Input: part model. Units: mm. Frame: model coordinates. Face numbers are marked on the shaded views. A direction names the side the tool comes from. Coordinates: 2 decimals unless noted, no trailing zeros. Order: outer loops, then holes, each group sorted by start corner. A loop starts at its lowest first (then second) coordinate and runs counter-clockwise, first axis right, second up. Notation, with made-up numbers: M -22,-2.75 L 35,-2.75 A17 cw 35,13.25 Z; hole C 36,-21 d6. An arc over 180 degrees is marked long. One line per item, written item: value.
Solid Edge part; units mm, degrees
sketch "Sketch1" plane through (0, 0, 0) normal (0, -1, 0) x (1, 0, 0)
  line L0 (7.5, -37.5) -> (-7.5, -37.5)
  line L1 (-7.5, -37.5) -> (-7.5, 47.5)
  line L2 (-7.5, 47.5) -> (-20.5, 47.5)
  line L3 (-20.5, 47.5) -> (-20.5, -47.5)
  line L4 (-20.5, -47.5) -> (20.5, -47.5)
  line L5 (20.5, -47.5) -> (20.5, 47.5)
  line L6 (20.5, 47.5) -> (7.5, 47.5)
  line L7 (7.5, 47.5) -> (7.5, -37.5)
extrude "Protrusion1" add sketch "Sketch1" against normal blind 33.5
fillet "Round1" radius 5 2 edges at (7.5, 16.75, -37.5) (-7.5, 16.75, -37.5)
fillet "Round2" radius 5 2 edges at (7.5, 16.75, 47.5) (-7.5, 16.75, 47.5)
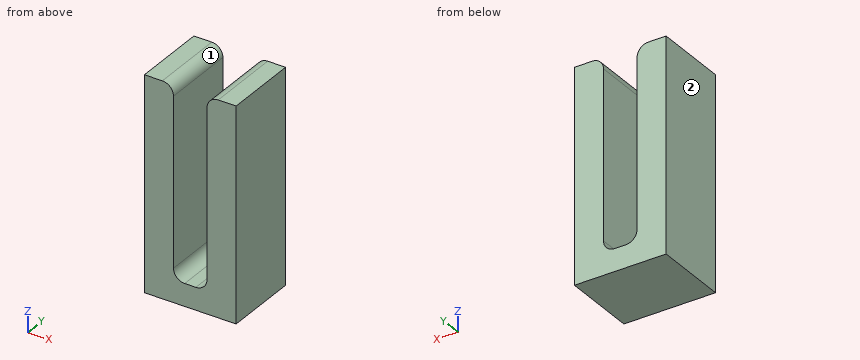
(1) Access query for the marked faces 1 and 2. Directions: +Z, -Z, +X, -X, +Y, -Y. A direction counts if a zero-diameter tool reaches every point of the face in a straight line with its end or side. Return the directions, or none.
Data:
face 1: +Z, +Y, -Y
face 2: +Z, -Z, -X, +Y, -Y
(2) Cut plane C-C on x = 4. Output: boundary loops of the cut face in (y, z), plus the area to 3 significant figures.
Data:
outline: M 0,-47.5 L 33.5,-47.5 L 33.5,-37.27 L 0,-37.27 Z
area: 343 mm2
(3) Cut plane B-B on y = 22. Output: boundary loops of the cut face in (x, z), plus the area to 3 significant figures.
Data:
outline: M -20.5,-47.5 L 20.5,-47.5 L 20.5,47.5 L 12.5,47.5 A5 ccw 7.5,42.5 L 7.5,-32.5 A5 cw 2.5,-37.5 L -2.5,-37.5 A5 cw -7.5,-32.5 L -7.5,42.5 A5 ccw -12.5,47.5 L -20.5,47.5 Z
area: 2,620 mm2
(4) First-contact query: pin 1 (1.5 mm diameter, centred on x = 0, y = 22.5, fed in from +Z); pin 2 (1.5 mm diameter, centred on x = -9, y = 16.5, fed in from +Z). Flat tips, straight axial feed; report the tip coordinate or a pass-through.
Data:
pin 1: stops at z = -37.5
pin 2: stops at z = 46.68
(5) Ray query, line 1 (X direction, y = 18, z = 18.5); line 2 (Z direction, x = 2, y = 18); line 3 (Z direction, x = -6, y = 13.5). Return the intervals inside material, ascending. Write a range as from..to.
Data:
line 1: x = -20.5..-7.5, 7.5..20.5
line 2: z = -47.5..-37.5
line 3: z = -47.5..-36.07
(6) Cut plane A-A on z = -8.5. Output: boundary loops of the cut face in (x, y), plus the area to 3 significant figures.
Data:
outline: M -20.5,0 L -7.5,0 L -7.5,33.5 L -20.5,33.5 Z; M 7.5,0 L 20.5,0 L 20.5,33.5 L 7.5,33.5 Z
area: 871 mm2
